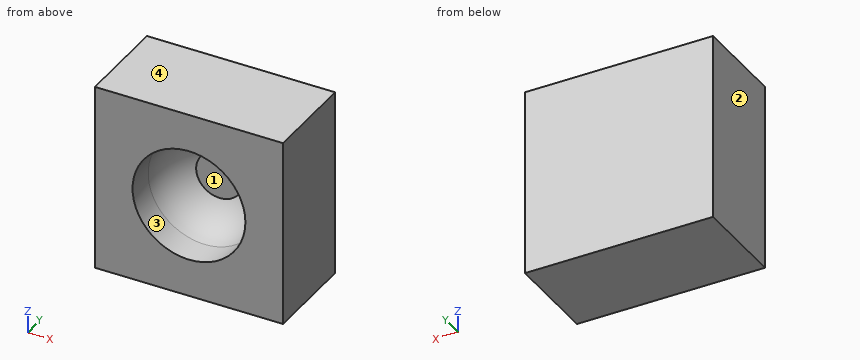
from build123d import *

# Parameters (mm, degrees)
SKETCH1_W           = 20
SKETCH1_H           = 20
BOSS_EXTRUDE1_DEPTH = 10


# Read off the part's stored shape, not the designer's step: Cavity1
with BuildPart() as part:
    # Sketch1 → Boss-Extrude1 (new body)
    with BuildSketch(Plane(origin=(0, 0, 0), x_dir=(1, 0, 0), z_dir=(0, 1, 0))):
        Rectangle(SKETCH1_W, SKETCH1_H)
    extrude(amount=BOSS_EXTRUDE1_DEPTH)

    # Cavity1 outline → Cavity1 (revolve, cut)
    with BuildSketch(Plane.XY):
        with BuildLine():
            Line((2.5, 5.9), (0, 5.9))
            Line((0, 5.9), (0, 0))
            Line((0, 0), (6, 0))
            Line((6, 0), (6, 3))
            ThreePointArc((6, 3), (4.909210346, 5.920864533), (2.5, 7.9))
            Line((2.5, 7.9), (2.5, 5.9))
        make_face()
    revolve(axis=Axis((0, 0, 0), (0, 1, 0)), mode=Mode.SUBTRACT)


solid = part.part
The listing builds one solid part. Answer for the finished solid, in the listing's coordinates (mm). Face numbers are marked on the shaded views. Coordinates: 2 decimals unless noted, no trailing zeros. Answer in a Markdown table with one row per item. Add a question column.
Item 1: Find section A-A (y = 7). State how many separate pieces and enclosed holes the cut face has, then the cut area to 3 significant figures.
Item 2: Find the intervals of material crossed by L1, parallel to X at y = 0.65, z = 0; L2, parallel to Z at x = -4, y = 1, in increasing order. Write a range as from..to.
Item 3: This flat-tipped pin is pushed along its axis until it touches: P1, Ø4, axis at x = -1, z = 1, coming from the -Y side. Where does it stop, or does it pass through?
Item 4: Determine the mould class of the marked faces 1, 2, 3 and 4 for opening direction X: +X half, -X half, draft (parallel to the pull), parting line (faces both ways), or undercut.
Result set:
| question | item | result |
|---|---|---|
| 1 | separate pieces | 2 |
| 1 | enclosed holes | 1 |
| 1 | area | 371 mm² |
| 2 | L1 | x = -10..-6, 6..10 |
| 2 | L2 | z = -10..-4.47, 4.47..10 |
| 3 | P1 | stops at y = 5.9 |
| 4 | face 1 | undercut |
| 4 | face 2 | -X half |
| 4 | face 3 | undercut |
| 4 | face 4 | draft |
